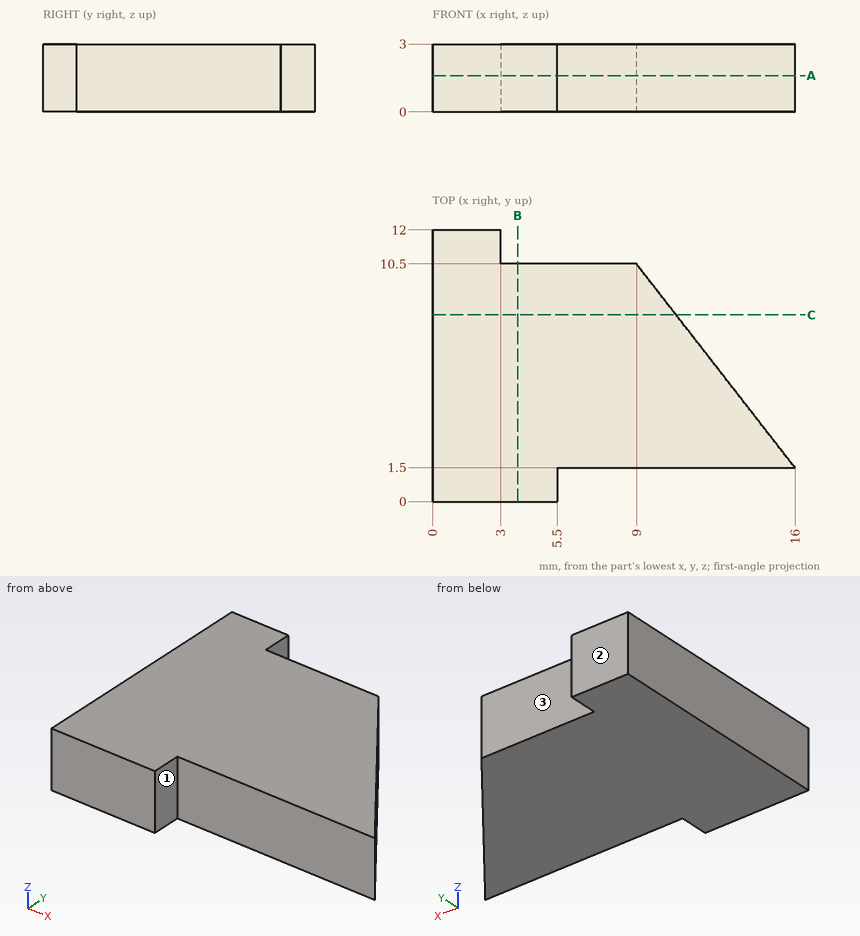
Verification items for this drawing (mm, ordinates from the low corner). A direction names the side the tool comes from. Coordinates: 2 decimals unless noted, no trailing zeros. Write each loop counter-clockwise with the first axis right and the second up, starting at its lowest first coordinate (ties: lowest second). Pieces come first, ordered by that corner, then holes. Notation, with made-up numbers: M -28.75,-14.5 L -14.75,-14.5 A16 cw -14.75,9.5 Z; hole C 76,56.25 d1. An arc over 180 degrees is marked long. One line per item, written item: value. Start each with the question number.
(1) Tool access check on the marked faces 1, 2 and 3. Record the directions out of +Z, -Z, +X, -X, +Y, -Y that give a thin tool (end or side, any length) a straight path to the whole face; none if there is none.
(2) Scan lines: line 1 along Y through (x, z) = (4.25, 0.3); line 2 along Y through (x, z) = (8, 0.25); line 3 along X through (y, z) = (2.75, 1.7). Record each from-to range of solid material in increasing order. Write a range as [from, to].
(3) Depth check by flat-ended pin: pin 1 (1.5 mm diameter, centred on x = 9.5, z = 0.5, fed in from -Y); pin 2 (1.6 mm diameter, centred on y = 1, z = 1.5, fed in from +X); pin 3 (0.8 mm diameter, centred on y = 11.5, z = 1, fed in from +X). Enter the tip coordinate at first touch or a pass-through.
(4) Sectioned sample at A-A, the plane z = 1.6. Enter the section's corners in (x, y), and give its area (3 significant figures).
(5) Sectioned sample at B-B, the plane x = 3.75. Enter the section's corners in (y, z), and give its area (3 significant figures).
(6) Sectioned sample at C-C, the plane y = 8.25. Enter the section's corners in (x, z).
Filled sheet:
1. face 1: +Z, -Z, +X, -Y
1. face 2: +Z, -Z, +X, -X, +Y
1. face 3: +Z, -Z, +X, +Y
2. line 1: [0, 10.5]
2. line 2: [1.5, 10.5]
2. line 3: [0, 15.03]
3. pin 1: y = 1.5
3. pin 2: x = 16
3. pin 3: x = 3
4. outline: M 0,0 L 5.5,0 L 5.5,1.5 L 16,1.5 L 9,10.5 L 3,10.5 L 3,12 L 0,12 Z
4. area: 125 mm²
5. outline: M 0,0 L 10.5,0 L 10.5,3 L 0,3 Z
5. area: 31.5 mm²
6. outline: M 0,0 L 10.75,0 L 10.75,3 L 0,3 Z
